```python
from build123d import *

# Parameters (mm, degrees)
F0_W     = 25.4
F0_H     = 25.4
F1_DEPTH = 25.4
F2_W     = 25.4
F2_H     = 25.4
F3_DEPTH = 25.4


with BuildPart() as f1:
    # F0 (on Front) → F1 (new body)
    with BuildSketch(Plane.XZ):
        with Locations((12.7, 12.7)):
            Rectangle(F0_W, F0_H)
        with Locations((-12.7, 12.7)):
            Rectangle(F0_W, F0_H)
        with Locations((12.7, -12.7)):
            Rectangle(F0_W, F0_H)
        with Locations((38.1, 12.7)):
            Rectangle(F0_W, F0_H)
        with Locations((38.1, -12.7)):
            Rectangle(F0_W, F0_H)
    extrude(amount=F1_DEPTH)

    # F2 (on Top) → F3 (join)
    with BuildSketch(Plane.XY):
        with Locations((12.7, 12.7)):
            Rectangle(F2_W, F2_H)
    extrude(amount=F3_DEPTH)


solid = f1.part
```
Work out the finished part from the listing and answer in its coordinate system (mm). A direction names the side the tool comes from. Give positions to 0.01 mm unless a question says otherwise; leave off trailing zeros. Order: outer loops, then holes, each group sorted by start corner. A loop starts at its lowest first (then second) coordinate and runs counter-clockwise, first axis right, second up.
1. Section B-B, the plane x = 6 is taken. Determine the outline of the cut face in (y, z).
Result sheet:
outline: (-25.4, -25.4) - (0, -25.4) - (0, 0) - (25.4, 0) - (25.4, 25.4) - (-25.4, 25.4) - close
2. For faces 1 (the flat face through (0, -13, -13)), 2 (the flat face through (25.4, 13, 13)), 3 (the flat face through (13, 13, 0)), determine the directions among +Z, -Z, +X, -X, +Y, -Y from which every point of the face is accessible in a straight line to the end or side of a thin tool.
Result sheet:
face 1: -Z, -X, +Y, -Y
face 2: +Z, -Z, +X, +Y
face 3: -Z, +X, -X, +Y
3. Straight lines are drawn through the part: L1, parallel to X at y = -4, z = -5.5; L2, parallel to X at y = 6, z = 6. For each, find the intervals that lie inside material, in ascending order.
Result sheet:
L1: x = 0 to 50.8
L2: x = 0 to 25.4
4. Section A-A, the plane z = 14.5 is taken. Determine the outline of the cut face in (x, y), and give its area (3 significant figures).
Result sheet:
outline: (-25.4, -25.4) - (50.8, -25.4) - (50.8, 0) - (25.4, 0) - (25.4, 25.4) - (0, 25.4) - (0, 0) - (-25.4, 0) - close
area: 2,580 mm2
5. Each of these flat-tipped pins is pushed along its axis until it touches: P1, Ø8, axis at y = 7, z = 20, coming from the +X side; P2, Ø12.5, axis at x = -11.5, z = 19, coming from the +Y side; P3, Ø7.5, axis at y = -17, z = -18, coming from the -X side. Where does it stop, or does it pass through?
Result sheet:
P1: stops at x = 25.4
P2: stops at y = 0
P3: stops at x = 0
6. Section D-D, the plane y = 15.5 is taken. Determine the outline of the cut face in (x, z), and give its area (3 significant figures).
Result sheet:
outline: (0, 0) - (25.4, 0) - (25.4, 25.4) - (0, 25.4) - close
area: 645 mm2
7. Section C-C, the plane y = -19 is taken. Determine the outline of the cut face in (x, z).
Result sheet:
outline: (-25.4, 0) - (0, 0) - (0, -25.4) - (50.8, -25.4) - (50.8, 25.4) - (-25.4, 25.4) - close
